CAD build for the part. Positions are in the model's coordinates, mm. A direction names the side the tool comes from. Round coordinates to 2 decimals unless told otherwise and drop trailing zeros. Order: outer loops, then holes, each group sorted by start corner. A loop starts at its lowest first (then second) coordinate and runs counter-clockwise, first axis right, second up. Notation, with made-up numbers: (24, 22.25) - (54, 22.25) arc R19 ccw to (54, 54.25) - close; hole circle Ø4 at (-18.5, -31). An arc over 180 degrees is marked (long way). Write item = value, one per line.
from build123d import *

# Parameters (mm, degrees)
SKETCH_1_W          = 100
SKETCH_1_H          = 60
EXTRUDE_1_DEPTH     = 40
SHELL_1_T           = -2
SKETCH_2_W          = 15
SKETCH_2_H          = 30
CUT_EXTRUDE_1_DEPTH = 60


with BuildPart() as part:
    # 草圖1 → 填料-伸長1 (new body)
    with BuildSketch(Plane.XY):
        Rectangle(SKETCH_1_W, SKETCH_1_H)
    extrude(amount=EXTRUDE_1_DEPTH)

    # 薄殼1
    shell_1_openings = [part.faces().sort_by_distance(p)[0] for p in [
        (0, 0, 40),
    ]]
    offset(amount=SHELL_1_T, openings=shell_1_openings, kind=Kind.INTERSECTION)

    # 草圖2 → 除料-伸長1 (cut)
    with BuildSketch(Plane.XZ.offset(30)):
        with Locations((-32.5, 25)):
            Rectangle(SKETCH_2_W, SKETCH_2_H)
    extrude(amount=-CUT_EXTRUDE_1_DEPTH, mode=Mode.SUBTRACT)


solid = part.part
(1) Probe line 1 along X through (y, z) = (-25.5, 12.5); line 2 along Y through (x, z) = (-17.5, 3); line 3 along Z through (x, y) = (13.5, 2). List the from-to ranges inside material, lowest first.
Solved:
line_1 = -50 to -48, 48 to 50
line_2 = -30 to -28, 28 to 30
line_3 = 0 to 2
(2) Band-saw the part on D-D on x = -38. List the corners of the cut face in (y, z).
Solved:
outline = (-30, 0) - (30, 0) - (30, 10) - (28, 10) - (28, 2) - (-28, 2) - (-28, 10) - (-30, 10) - close
(3) Drop flat-ended pins along their axis: pin 1 (1 mm diameter, centred on x = -30.5, y = -28.5, fed in from +Z); pin 2 (10 mm diameter, centred on x = -22, y = -9, fed in from +Z). Give the stop position or say it passes through.
Solved:
pin_1 = 10
pin_2 = 2
(4) Band-saw the part on C-C on y = 15.5. List the corners of the cut face in (x, z).
Solved:
outline = (-50, 0) - (50, 0) - (50, 40) - (48, 40) - (48, 2) - (-48, 2) - (-48, 40) - (-50, 40) - close
(5) Pull direction Y, two halves, no side cores. Call faces 1 (the flat face through (-1, 0, 2)), 2 (the flat face through (-1, 0, 0)), 3 (the flat face through (-1, -30, 20)), 4 (the flat face through (-1, 30, 20)): released by +Y, released by -Y, zero draft, split by the parting line, or undercut.
Solved:
face_1 = undercut
face_2 = zero draft
face_3 = released by -Y
face_4 = released by +Y
(6) Band-saw the part on B-B on z = 37. List the corners of the cut face in (x, y), plus the area to 3 significant figures.
Solved:
outline = (-50, -30) - (-40, -30) - (-40, -28) - (-48, -28) - (-48, 28) - (-40, 28) - (-40, 30) - (-50, 30) - close; (-25, -30) - (50, -30) - (50, 30) - (-25, 30) - (-25, 28) - (48, 28) - (48, -28) - (-25, -28) - close
area = 564 mm²
(7) Tool access for faces 5 (the flat face through (-48.4, 6.8, 40)), 6 (the flat face through (-40, 29, 25)), 7 (the flat face through (-1, -28, 21)): list every direction of +Z, -Z, +X, -X, +Y, -Y with a clear straight run to the whole face (end or side of a thin tool).
Solved:
face_5 = +Z, +X, -X, +Y, -Y
face_6 = +Z, +Y, -Y
face_7 = +Z
(8) Band-saw the part on A-A on z = 8. List the corners of the cut face in (x, y).
Solved:
outline = (-50, -30) - (50, -30) - (50, 30) - (-50, 30) - close; hole (-48, -28) - (48, -28) - (48, 28) - (-48, 28) - close
